```python
from build123d import *

# Parameters (mm, degrees)
PANEL_DEPTH                 = 0.79
SKETCH3_R                   = 1.125
OUTER_HINGE_MOUNT_DEPTH     = 0.79
SKETCH4_R                   = 2.25
MOUNTING_PLATE_HOLES_DEPTH  = 10
SKETCH7_R                   = 1.125
NEW_INNER_HINGE_MOUNT_DEPTH = 10


with BuildPart() as part:
    # Sketch1 → Panel (new body)
    with BuildSketch(Plane(origin=(0, 0, 0), x_dir=(1, 0, 0), z_dir=(0, 1, 0))):
        Polygon((65.326251897, 149.069802731), (95.326251897, 149.069802731), (95.326251897, -183.930197269), (-94.673748103, -183.930197269), (-94.673748103, 149.069802731), (-64.673748103, 149.069802731), (-64.673748103, 156.069802731), (-39.673748103, 156.069802731), (-39.673748103, 149.069802731), (40.326251897, 149.069802731), (40.326251897, 156.069802731), (65.326251897, 156.069802731), align=None)
    extrude(amount=PANEL_DEPTH)

    # Sketch3 → Outer Hinge Mount (cut)
    with BuildSketch(Plane(origin=(0, 0.79, 0), x_dir=(1, 0, 0), z_dir=(0, 1, 0))):
        with Locations(Location((-88.673748103, -112.930197269, 0), (0, 0, 270))):
            Circle(SKETCH3_R)
        with Locations(Location((-88.673748103, -129.930197269, 0), (0, 0, 270))):
            Circle(SKETCH3_R)
        with BuildLine():
            Line((-94.673748103, -108.930197269), (-93.673748103, -108.930197269))
            ThreePointArc((-93.673748103, -108.930197269), (-93.320194713, -109.076643878), (-93.173748103, -109.430197269))
            Line((-93.173748103, -109.430197269), (-93.173748103, -133.430197269))
            ThreePointArc((-93.173748103, -133.430197269), (-93.320194713, -133.783750659), (-93.673748103, -133.930197269))
            Line((-93.673748103, -133.930197269), (-94.673748103, -133.930197269))
            Line((-94.673748103, -133.930197269), (-94.673748103, -108.930197269))
        make_face()
    outer_hinge_mount = extrude(amount=-OUTER_HINGE_MOUNT_DEPTH, mode=Mode.SUBTRACT)

    # Mirror1: Outer Hinge Mount across plane
    add(outer_hinge_mount.mirror(Plane.XY.offset(13.930197269)), mode=Mode.SUBTRACT)

    # Sketch4 → Mounting Plate Holes (cut)
    with BuildSketch(Plane(origin=(0, 0.79, 0), x_dir=(1, 0, 0), z_dir=(0, 1, 0))):
        with Locations(Location((-31.176486576, 17.572541204, 0), (0, 0, 270))):
            Circle(SKETCH4_R)
        with Locations(Location((31.82899037, 17.572541204, 0), (0, 0, 270))):
            Circle(SKETCH4_R)
        with Locations(Location((31.82899037, -45.432935741, 0), (0, 0, 270))):
            Circle(SKETCH4_R)
        with Locations(Location((-31.176486576, -45.432935741, 0), (0, 0, 270))):
            Circle(SKETCH4_R)
    extrude(amount=-MOUNTING_PLATE_HOLES_DEPTH, mode=Mode.SUBTRACT)

    # Sketch7 → New Inner Hinge Mount (cut)
    with BuildSketch(Plane(origin=(0, 0.79, 0), x_dir=(1, 0, 0), z_dir=(0, 1, 0))):
        with Locations(Location((89.326251897, -111.430197269, 0), (0, 0, 270))):
            Circle(SKETCH7_R)
        with Locations(Location((89.326251897, -131.430197269, 0), (0, 0, 270))):
            Circle(SKETCH7_R)
        with BuildLine():
            Line((95.326251897, -108.930197269), (94.246251897, -108.930197269))
            ThreePointArc((94.246251897, -108.930197269), (93.892698506, -109.076643878), (93.746251897, -109.430197269))
            Line((93.746251897, -109.430197269), (93.746251897, -133.296285761))
            ThreePointArc((93.746251897, -133.296285761), (93.931920279, -133.744528887), (94.380163405, -133.930197269))
            Line((94.380163405, -133.930197269), (95.326251897, -133.930197269))
            Line((95.326251897, -133.930197269), (95.326251897, -108.930197269))
        make_face()
    new_inner_hinge_mount = extrude(amount=-NEW_INNER_HINGE_MOUNT_DEPTH, mode=Mode.SUBTRACT)

    # Mirror3: New Inner Hinge Mount across plane
    add(new_inner_hinge_mount.mirror(Plane.XY.offset(13.930197269)), mode=Mode.SUBTRACT)


solid = part.part
```
Check sheet for the modelled part. Datum: model origin and axes. Units: mm. Coordinates: 2 decimals unless noted, no trailing zeros. Write each loop counter-clockwise with the first axis right and the second up, starting at its lowest first coordinate (ties: lowest second). Pieces come first, ordered by that corner, then holes. Notation, with made-up numbers: (-26, 39.5) -> (16, 39.5) arc R20 ccw to (16, 75.5) -> close; hole circle Ø5 at (-1, -27). An arc over 180 degrees is marked (long way). Use a Markdown table: item, result.
1. Sectioned sample at A-A (x = 6). Enter the section's corners in (y, z).
Reported:
| item | result |
|---|---|
| outline | (0, -149.07) -> (0.79, -149.07) -> (0.79, 183.93) -> (0, 183.93) -> close |
2. Sectioned sample at B-B (y = 0.25). Give the number of separate pieces and of enclosed holes in the cut face, plus the area to 3 significant figures.
Reported:
| item | result |
|---|---|
| separate pieces | 1 |
| enclosed holes | 12 |
| area | 63,400 mm2 |
3. Scan lines: line 1 along X through (y, z) = (0.65, 46); line 2 along Z through (x, y) = (-5, 0.55); line 3 along X through (y, z) = (0.1, -93). Record each from-to range of solid material in increasing order.
Reported:
| item | result |
|---|---|
| line 1 | x = -94.67 to -33.35, -29 to 29.65, 34.01 to 95.33 |
| line 2 | z = -149.07 to 183.93 |
| line 3 | x = -93.17 to 93.75 |
4. Sectioned sample at C-C (z = -96). Enter the section's corners in (x, y), plus the area to 3 significant figures.
Reported:
| item | result |
|---|---|
| outline | (-93.17, 0) -> (93.75, 0) -> (93.75, 0.79) -> (-93.17, 0.79) -> close |
| area | 148 mm2 |
